Check sheet for the drawn part. Datum: minimum x, y, z corner. Units: mm. A direction names the side the tool comes from. Give positions to 0.01 mm unless a question says otherwise; leave off trailing zeros. Loops run counter-clockwise (first coordinate to the right, second up) from the corner with the lowest first, then second, coordinate; pieces in that order, holes last. Notation, with made-up numbers: M 34.5,24.25 L 88.5,24.25 A32 cw 88.5,50.25 Z; hole C 66,80.5 d9. An arc over 180 degrees is marked long. Write each question's results on one line, items separated by ' | '. Start each with the question number.
1. Tool access check on the marked faces 1 and 2. Record the directions out of +Z, -Z, +X, -X, +Y, -Y that give a thin tool (end or side, any length) a straight path to the whole face; none if there is none.
2. Draft check along X on the marked faces 3, 4 and 5. Enter one of: pulls with the +X half, pulls with the -X half, needs draft (parallel to the pull), parting line crosses it, or undercut.
3. Sectioned sample at A-A on z = 280. Record the cut outline in (x, y).
4. Go/stop test with a flat-tipped pin: pin 1 (7 mm diameter, centred on y = 2.5, z = 193.5, fed in from -X). Record where the tip stops, or that it passes through.
5. Sectioned sample at B-B on x = 165.1. Record the cut outline in (y, z).
6. Sectioned sample at C-C on y = 61. Record the cut outline in (x, z).
7. Material ranges on line 1 along Y through (x, z) = (48, 253); line 2 along X through (y, z) = (74, 250); line 3 along Z through (x, y) = (226.5, 69.5), recorded low to high.
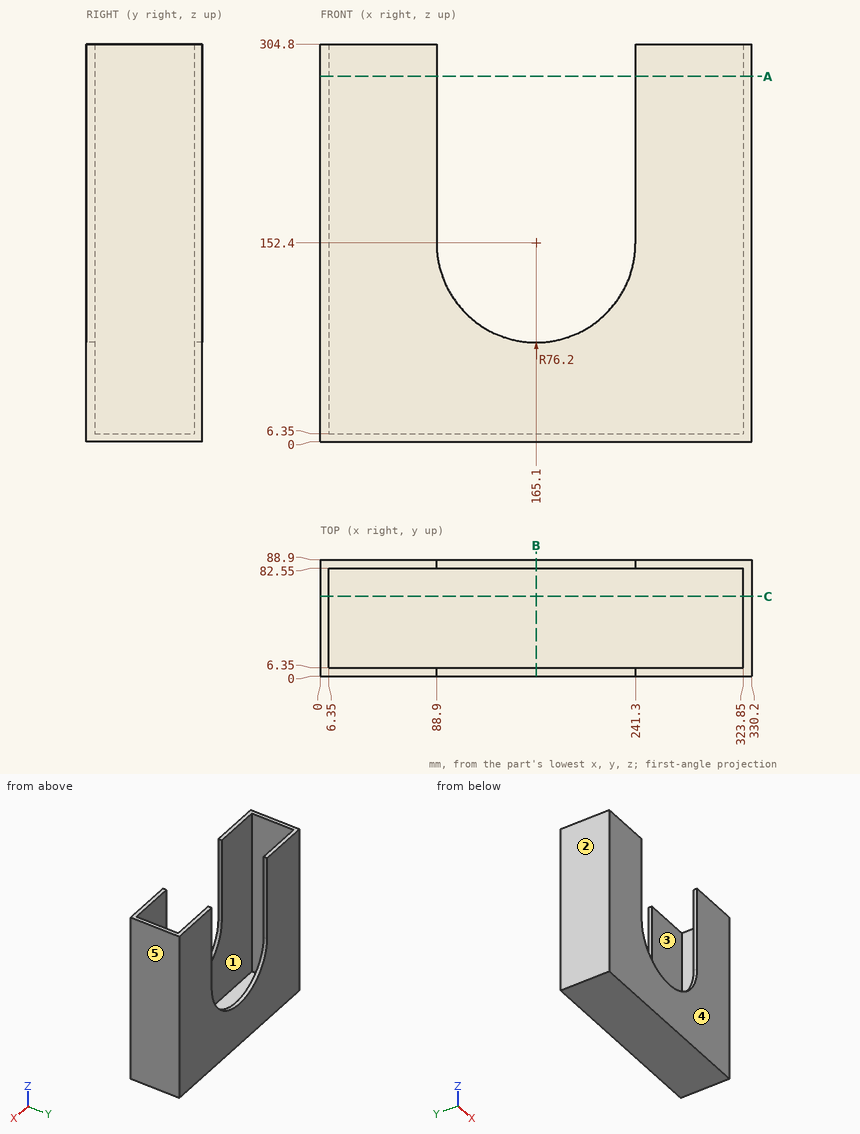
Output values:
1) face 1: +Z | face 2: +Z, -Z, -X, +Y, -Y
2) face 3: undercut | face 4: needs draft | face 5: pulls with the +X half
3) outline: M 0,0 L 88.9,0 L 88.9,6.35 L 6.35,6.35 L 6.35,82.55 L 88.9,82.55 L 88.9,88.9 L 0,88.9 Z; M 241.3,0 L 330.2,0 L 330.2,88.9 L 241.3,88.9 L 241.3,82.55 L 323.85,82.55 L 323.85,6.35 L 241.3,6.35 Z
4) pin 1: x = 0
5) outline: M 0,0 L 88.9,0 L 88.9,76.2 L 82.55,76.2 L 82.55,6.35 L 6.35,6.35 L 6.35,76.2 L 0,76.2 Z
6) outline: M 0,0 L 330.2,0 L 330.2,304.8 L 323.85,304.8 L 323.85,6.35 L 6.35,6.35 L 6.35,304.8 L 0,304.8 Z
7) line 1: 0 to 6.35, 82.55 to 88.9 | line 2: 0 to 6.35, 323.85 to 330.2 | line 3: 0 to 6.35
